The drawing under review shows one solid part. Ordinate dimensions are in mm from its lowest x, y, z. Round coordinates to 2 decimals unless told otherwise and drop trailing zeros. Order: outer loops, then holes, each group sorted by start corner. A loop starts at its lowest first (then second) coordinate and runs counter-clockwise, first axis right, second up. Notation, with made-up numbers: M -29.75,71.5 L -5.75,71.5 A14 cw -5.75,76.5 Z; hole C 7.5,22 d3. An arc over 180 degrees is marked long. Use a Markdown table: item, result.
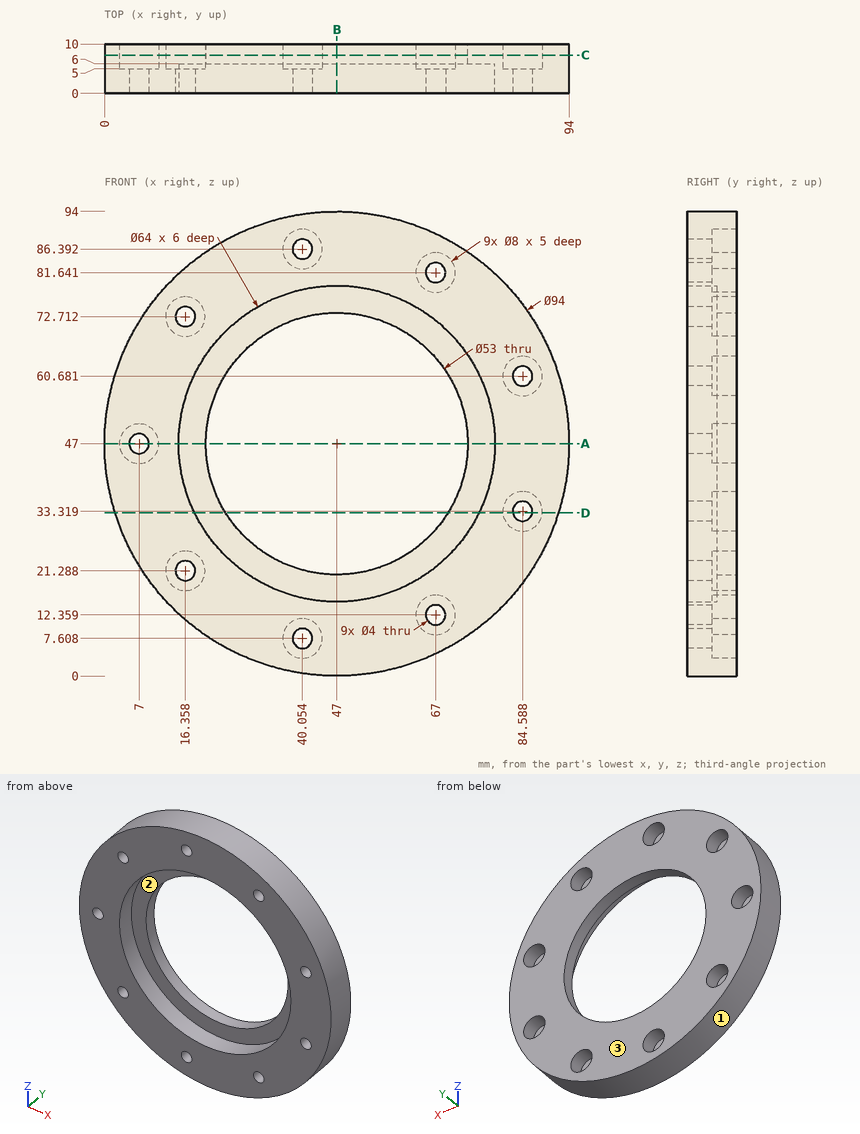
Q1. Clearance check with flat-ended pins moving along their axes: pin 1 (4.5 mm diameter, centred on x = 84.59, z = 33.32, fed in from -Y); pin 2 (2.5 mm diameter, centred on x = 8, z = 46.5, fed in from +Y); pin 3 (5 mm diameter, centred on x = 45, y = 8, fed in from -Z); pin 4 (2 mm diameter, centred on x = 74.5, y = 3.5, fed in from -Z). State where each tip first meets the part, or that it passes through.
Determined:
| item | result |
|---|---|
| pin 1 | stops at y = 0 |
| pin 2 | stops at y = 5 |
| pin 3 | stops at z = 0 |
| pin 4 | stops at z = 8.18 |
Q2. Add section A-A (z = 47). Write out the cut boundary in (x, y), then the cut area to 3 significant figures.
Determined:
| item | result |
|---|---|
| outline | M 0,0 L 5,0 L 5,5 L 3,5 L 3,10 L 0,10 Z; M 9,0 L 15,0 L 15,6 L 20.5,6 L 20.5,10 L 11,10 L 11,5 L 9,5 Z; M 73.5,6 L 79,6 L 79,0 L 94,0 L 94,10 L 73.5,10 Z |
| area | 284 mm^2 |
Q3. Add section B-B (x = 47). Write out the cut boundary in (y, z).
Determined:
| item | result |
|---|---|
| outline | M 0,0 L 10,0 L 10,20.5 L 6,20.5 L 6,15 L 0,15 Z; M 0,79 L 6,79 L 6,73.5 L 10,73.5 L 10,94 L 0,94 Z |
Q4. Draft analysis for pull direction Z (two halves, no side actions). For the marked faces 1, 2 and 3, state which applies: pulls with the +Z half, pulls with the -Z half, needs draft (parallel to the pull), parting line crosses it, or undercut.
Determined:
| item | result |
|---|---|
| face 1 | parting line crosses it |
| face 2 | undercut |
| face 3 | needs draft |
Q5. Add section D-D (z = 33). Write out the cut boundary in (x, y) (1 decimal).
Determined:
| item | result |
|---|---|
| outline | M 2.1,0 L 18.2,0 L 18.2,6 L 24.5,6 L 24.5,10 L 2.1,10 Z; M 69.5,6 L 75.8,6 L 75.8,0 L 82.6,0 L 82.6,5 L 80.6,5 L 80.6,10 L 69.5,10 Z; M 86.6,0 L 91.9,0 L 91.9,10 L 88.6,10 L 88.6,5 L 86.6,5 Z |
Q6. Wall thickness on line 1 along Z through (x, y) = (85, 7) (1 decimal); line 2 along X through (y, z) = (1.75, 34) (1 decimal); line 3 along Z through (x, y) = (47, 7.3): over which ranges is each line inside the solid? List them lowest first. Write a range as [from, to].
Determined:
| item | result |
|---|---|
| line 1 | z = [19.3, 29.3], [37.3, 56.7], [64.7, 74.7] |
| line 2 | x = [1.8, 17.8], [76.2, 82.7], [86.5, 92.2] |
| line 3 | z = [0, 20.5], [73.5, 94] |
Q7. Add section C-C (y = 7.75). Give the number of separate pieces and of enclosed holes in the cut face, then the cut area to 3 significant figures.
Determined:
| item | result |
|---|---|
| separate pieces | 1 |
| enclosed holes | 10 |
| area | 4,280 mm^2 |
